Part model, mm, in its own coordinate system. A direction names the side the tool comes from. Coordinates: 2 decimals unless noted, no trailing zeros. Write each loop counter-clockwise with the first axis right and the second up, starting at its lowest first coordinate (ties: lowest second). Pieces come first, ordered by that corner, then holes. Notation, with made-up numbers: M 2,34.5 L 47,34.5 A27 cw 47,51.5 Z; hole C 89,3 d11. An arc over 180 degrees is marked long. Use a Markdown table: item, result. Add a question column.
Q1. Wall check: L1, parallel to Z at x = 0, y = 76; L2, parallel to X at y = 35, z = 22. Give the ranges that are in metal, low to high. Write a range as from..to.
Q2. Mould opens along X. For faces 4 (the cylindrical face through (-32.907, 87.508, -10.363)), 5 (the cylindrical face through (18.28, 199.86, 28.67)), 6 (the flat face through (25.03, 210, 22.51)) say: released by +X, released by -X, zero draft, split by the parting line, or undercut.
Q3. Pin check, flat tips, straight feed: pin 1 Ø3 at (x, y) = (1.5, 92.5) entering from -Z; pin 2 Ø5 at (x, y) = (-15.5, 135) entering from -Z; pin 3 Ø1.8 at (y, z) = (200, 0) entering from -X. Stop position of each tip, or through.
Q4. Slice it at B-B on z = -17. Write the cut outline in (x, y), then the cut area to 3 significant figures.
Q5. Tool access for faces 1 (the flat face through (-5, 190, 34)), 2 (the cylindrical face through (-7.262, 193.522, -32.703)), 3 (the flat face through (-5.3, 177.5, 33.4)): list every direction of +Z, -Z, +X, -X, +Y, -Y with a clear straight run to the whole face (end or side of a thin tool).
Q6. Slice it at C-C on y = 116. Write the cut outline in (x, z), then the cut area to 3 significant figures.
Q7. Slice it at A-A on x = 0. Write the cut outline in (y, z).
Autodesk Inventor part; units mm, degrees
ref_plane "Work Plane2" through (35, 0, 0) normal (1, 0, 0) x (0, 1, 0)
ref_plane "Work Plane4" through (34, 0, 0) normal (1, 0, 0) x (0, 1, 0)
ref_plane "XZ Plane" through (0, 0, 0) normal (0, 1, 0) x (-1, 0, 0)
sketch "Sketch1" plane through (0, 0, 0) normal (0, 1, 0) x (-1, 0, 0)
  circle A0 centre (0, 0) radius 35
  circle A1 centre (0, 0) radius 34.5
  dimension "d0" = 70
  dimension "d1" = 69
extrude "Extrusion1" add sketch "Sketch1" along normal blind 190
ref_plane "Work Plane2" through (35, 0, 0) normal (1, 0, 0) x (0, 1, 0)
sketch "Sketch4" plane through (35, 0, 0) normal (1, 0, 0) x (0, 1, 0)
  line L0 (190, -35) -> (190, 35)
  point P0 (0, 0)
  point P1 (10, 0)
  dimension "d48" = 10
hole "Hole2" at (35, 10, 0) direction (-1, 0, 0) diameter 3 depth 8 tip angle 118
sketch "Sketch5" plane through (0, 190, 0) normal (0, 1, 0) x (1, 0, 0)
  circle A0 centre (0, 0) radius 34
  circle A1 centre (0, 0) radius 33.5
  dimension "d44" = 68
  dimension "d45" = 67
extrude "Extrusion3" add sketch "Sketch5" along normal blind 20
sketch "Sketch6" plane through (0, 190, 0) normal (0, -1, 0) x (1, 0, 0)
  circle A0 centre (0, 0) radius 33.5
  circle A1 centre (0, 0) radius 34.5
  circle A2 centre (0, 0) radius 35
extrude "Extrusion4" add sketch "Sketch6" along normal blind 12.5 contours A1
ref_plane "Work Plane4" through (34, 0, 0) normal (1, 0, 0) x (0, 1, 0)
sketch "Sketch8" plane through (34, 0, 0) normal (1, 0, 0) x (0, 1, 0)
  line L0 (210, -34) -> (210, 34)
  point P0 (0, 0)
  point P1 (200, 0)
  dimension "d61" = 10
hole "Hole4" at (34, 200, 0) direction (-1, 0, 0) diameter 3 depth 8 tip angle 118
pattern_circular "Circular Pattern2" count 3 over 360 about axis through (0, 0, 0) along (0, 1, 0) of "Hole2", "Hole4"
properties part number "Lower skin" material "Plastic, Opaque White"
Recorded:
| question | item | result |
|---|---|---|
| 1 | L1 | -35..-34.5, 34.5..35 |
| 1 | L2 | -27.22..-26.58, 26.58..27.22 |
| 2 | face 4 | undercut |
| 2 | face 5 | split by the parting line |
| 2 | face 6 | zero draft |
| 3 | pin 1 | z = -35 |
| 3 | pin 2 | z = -32.5 |
| 3 | pin 3 | x = -34 |
| 4 | outline | M -30.59,0 L -30.02,0 L -30.02,177.5 L -28.87,177.5 L -28.87,210 L -29.44,210 L -29.44,190 L -30.59,190 Z; M 28.87,177.5 L 30.02,177.5 L 30.02,0 L 30.59,0 L 30.59,190 L 29.44,190 L 29.44,210 L 28.87,210 Z |
| 4 | area | 270 mm² |
| 5 | face 1 | +Y |
| 5 | face 2 | +Y, -Y |
| 5 | face 3 | -Y |
| 6 | outline | C 0,0 d70; hole C 0,0 d69 |
| 6 | area | 109 mm² |
| 7 | outline | M 0,-35 L 190,-35 L 190,-34 L 210,-34 L 210,-33.5 L 177.5,-33.5 L 177.5,-34.5 L 0,-34.5 Z; M 0,34.5 L 177.5,34.5 L 177.5,33.5 L 210,33.5 L 210,34 L 190,34 L 190,35 L 0,35 Z |
